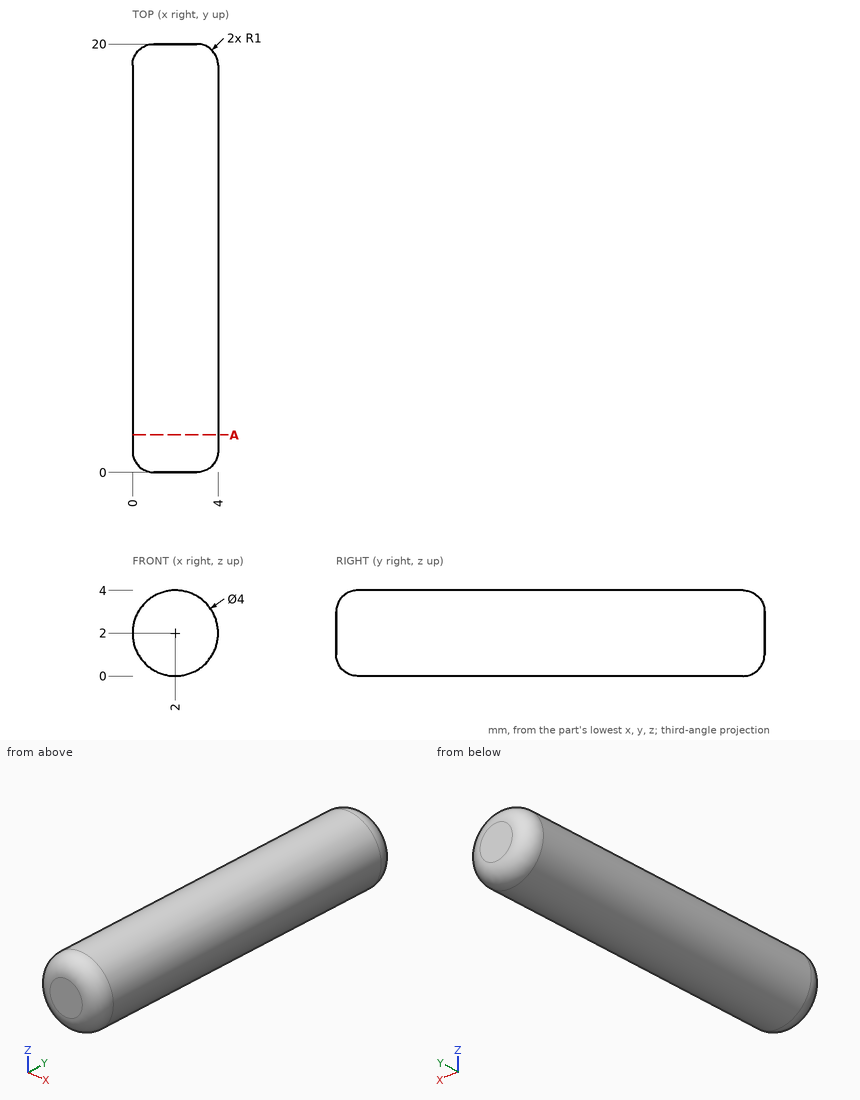
Design review of the part shown in the three views and the two pictorial views. Dimensions are in mm from the part's minimum x, y and z. Round coordinates to 2 decimals unless told otherwise and drop trailing zeros. Write each loop counter-clockwise with the first axis right and the second up, starting at its lowest first coordinate (ties: lowest second). Pieces come first, ordered by that corner, then holes. Notation, with made-up numbers: (26, -7) -> (32, -7) arc R28 cw to (32, 31) -> close; hole circle Ø2 at (60.25, 66.25). An arc over 180 degrees is marked (long way). Write item = value, one per line. Start each with the question number.
1) Wall thickness on probe 1 along Y at (x, z) = (1.2, 3.75); probe 2 along X at (y, z) = (4.5, 2.2); probe 3 along Z at (x, y) = (1.15, 9): over which ranges is each line inside the solid? List them lowest first. Write a range as from..to.
2) Take a section at A-A, the plane y = 1.75. State the section outline as (x, z) points, plus the area to 3 significant figures.
3) Clearance check with flat-ended pins moving along their axes: pin 1 (1.5 mm diameter, centred on x = 3.5, y = 15, fed in from +Z); pin 2 (1 mm diameter, centred on y = 8.5, z = 2.5, fed in from +X); pin 3 (1 mm diameter, centred on y = 7, z = 0.5, fed in from -X). State where each tip first meets the part, or that it passes through.
Results list:
q1.probe_1 = 0.62..19.38
q1.probe_2 = 0.01..3.99
q1.probe_3 = 0.19..3.81
q2.outline = circle Ø4 at (2, 2)
q2.area = 12.6 mm²
q3.pin_1 = 3.85
q3.pin_2 = 4
q3.pin_3 = 0.27
